Geometry check sheet. Reference: the model listing, model coordinates, mm. Coordinates: 2 decimals unless noted, no trailing zeros. One line per item, written item: value.
Autodesk Inventor part; units mm, degrees
ref_plane "YZ Plane" through (0, 0, 0) normal (1, 0, 0) x (0, 1, 0)
ref_plane "XZ Plane" through (0, 0, 0) normal (0, 1, 0) x (-1, 0, 0)
ref_plane "XY Plane" through (0, 0, 0) normal (0, 0, 1) x (1, 0, 0)
sketch "T-Slot 4040 Base" plane through (0, 0, 0) normal (0, 0, 1) x (1, 0, 0)
  line L0 (-28, 0) -> (28, 0) construction
  line L1 (0, -28) -> (0, 28) construction
  circle A0 centre (0, 0) radius 5.1
  line L2 (-7.5, -7.5) -> (7.5, -7.5)
  line L3 (7.5, -7.5) -> (7.5, 7.5)
  line L4 (7.5, 7.5) -> (-7.5, 7.5)
  line L5 (-7.5, 7.5) -> (-7.5, -7.5)
  line L6 (-7.5, -7.5) -> (7.5, 7.5) construction
  line L7 (7.5, -7.5) -> (-7.5, 7.5) construction
  line L8 (-20, 20) -> (20, 20)
  line L9 (20, 20) -> (20, -20)
  line L10 (20, -20) -> (-20, -20)
  line L11 (-20, -20) -> (-20, 20)
  line L12 (-20, 20) -> (20, -20) construction
  line L13 (20, 20) -> (-20, -20) construction
  line L14 (20, 5) -> (14.5, 5)
  line L15 (14.5, 5) -> (14.5, 10)
  line L16 (14.5, 10) -> (12.4749, 10)
  line L17 (12.4749, 10) -> (7.5, 5.0251)
  line L18 (5, 20) -> (5, 14.5)
  line L19 (5, 14.5) -> (10, 14.5)
  line L20 (10, 14.5) -> (10, 12.4749)
  line L21 (10, 12.4749) -> (5.0251, 7.5)
  line L22 (18.5, 18.5) -> (11.5, 18.5)
  line L23 (11.5, 18.5) -> (11.5, 11.5)
  line L24 (11.5, 11.5) -> (18.5, 11.5)
  line L25 (18.5, 11.5) -> (18.5, 18.5)
  line L26 (18.5, 18.5) -> (11.5, 11.5) construction
  line L27 (11.5, 18.5) -> (18.5, 11.5) construction
  line L28 (3.0732, 1.3088) -> (4.38, 2.6125) construction
  line L29 (5.905, 4.1338) -> (4.1393, 5.9037)
  line L30 (4.1393, 5.9037) -> (2.6122, 4.3802)
  line L31 (1.3075, 3.0787) -> (3.0732, 1.3088) construction
  line L32 (3.0732, 1.3088) -> (4.1393, 5.9037) construction
  line L33 (5.905, 4.1338) -> (1.3075, 3.0787) construction
  line L34 (4.38, 2.6125) -> (5.905, 4.1338)
  line L35 (2.6122, 4.3802) -> (1.3075, 3.0787) construction
  line L36 (-20, 5) -> (-14.5, 5)
  line L37 (-14.5, 5) -> (-14.5, 10)
  line L38 (-14.5, 10) -> (-12.4749, 10)
  line L39 (-12.4749, 10) -> (-7.5, 5.0251)
  line L40 (-5, 20) -> (-5, 14.5)
  line L41 (-5, 14.5) -> (-10, 14.5)
  line L42 (-10, 14.5) -> (-10, 12.4749)
  line L43 (-10, 12.4749) -> (-5.0251, 7.5)
  line L44 (-18.5, 18.5) -> (-11.5, 18.5)
  line L45 (-11.5, 18.5) -> (-11.5, 11.5)
  line L46 (-11.5, 11.5) -> (-18.5, 11.5)
  line L47 (-18.5, 11.5) -> (-18.5, 18.5)
  line L48 (-5.905, 4.1338) -> (-4.1393, 5.9037)
  line L49 (-4.1393, 5.9037) -> (-2.6122, 4.3802)
  line L50 (-4.38, 2.6125) -> (-5.905, 4.1338)
  line L51 (7.5, -7.5) -> (-7.5, -7.5)
  line L52 (20, -5) -> (14.5, -5)
  line L53 (14.5, -5) -> (14.5, -10)
  line L54 (14.5, -10) -> (12.4749, -10)
  line L55 (12.4749, -10) -> (7.5, -5.0251)
  line L56 (5, -20) -> (5, -14.5)
  line L57 (5, -14.5) -> (10, -14.5)
  line L58 (10, -14.5) -> (10, -12.4749)
  line L59 (10, -12.4749) -> (5.0251, -7.5)
  line L60 (18.5, -18.5) -> (11.5, -18.5)
  line L61 (11.5, -18.5) -> (11.5, -11.5)
  line L62 (11.5, -11.5) -> (18.5, -11.5)
  line L63 (18.5, -11.5) -> (18.5, -18.5)
  line L64 (18.5, -18.5) -> (11.5, -11.5) construction
  line L65 (11.5, -18.5) -> (18.5, -11.5) construction
  line L66 (3.0732, -1.3088) -> (4.38, -2.6125) construction
  line L67 (5.905, -4.1338) -> (4.1393, -5.9037)
  line L68 (4.1393, -5.9037) -> (2.6122, -4.3802)
  line L69 (1.3075, -3.0787) -> (3.0732, -1.3088) construction
  line L70 (3.0732, -1.3088) -> (4.1393, -5.9037) construction
  line L71 (5.905, -4.1338) -> (1.3075, -3.0787) construction
  line L72 (4.38, -2.6125) -> (5.905, -4.1338)
  line L73 (2.6122, -4.3802) -> (1.3075, -3.0787) construction
  line L74 (-4.38, -2.6125) -> (-5.905, -4.1338)
  line L75 (-4.1393, -5.9037) -> (-2.6122, -4.3802)
  line L76 (-5.905, -4.1338) -> (-4.1393, -5.9037)
  line L77 (-12.4749, -10) -> (-7.5, -5.0251)
  line L78 (-10, -12.4749) -> (-5.0251, -7.5)
  line L79 (-10, -14.5) -> (-10, -12.4749)
  line L80 (-5, -14.5) -> (-10, -14.5)
  line L81 (-5, -20) -> (-5, -14.5)
  line L82 (-18.5, -18.5) -> (-11.5, -18.5)
  line L83 (-11.5, -18.5) -> (-11.5, -11.5)
  line L84 (-11.5, -11.5) -> (-18.5, -11.5)
  line L85 (-18.5, -11.5) -> (-18.5, -18.5)
  line L86 (-14.5, -10) -> (-12.4749, -10)
  line L87 (-14.5, -5) -> (-14.5, -10)
  line L88 (-20, -5) -> (-14.5, -5)
  point P0 (15, 15)
  point P1 (3.6062, 3.6062)
  point P2 (3.6062, 3.6062)
  point P3 (15, -15)
  point P4 (3.6062, -3.6062)
  point P5 (3.6062, -3.6062)
  dimension "d9" = 10.2
  dimension "d12" = 40
  dimension "d13" = 40
  dimension "d14" = 5.5
  dimension "d15" = 15
  dimension "d16" = 7
  dimension "d17" = 10
  dimension "d20" = 1.75
  dimension "d21" = 7
  dimension "d22" = 2
  dimension "d29" = 1.5
  dimension "d30" = 2.5
extrude "Extrusion1" add sketch "T-Slot 4040 Base" along normal blind 500 contours L5 L4 L3 L2 | L2 L78 L79 L80 L81 L10 L11 L88 L87 L86 L77 L5 | L2 L3 L55 L54 L53 L52 L9 L10 L56 L57 L58 L59 | L39 L38 L37 L36 L11 L8 L40 L41 L42 L43 L4 L5 | L3 L4 L21 L20 L19 L18 L8 L9 L14 L15 L16 L17
fillet "Rundung1" radius 1 16 edges at (11.5, 18.5, 250) (18.5, 18.5, 250) (18.5, 11.5, 250) (11.5, 11.5, 250) (-11.5, 18.5, 250) (-18.5, 18.5, 250) (-18.5, 11.5, 250) (-11.5, 11.5, 250) (-18.5, -11.5, 250) (-11.5, -11.5, 250) (-11.5, -18.5, 250) (-18.5, -18.5, 250) (11.5, -18.5, 250) (11.5, -11.5, 250) (18.5, -11.5, 250) (18.5, -18.5, 250)
fillet "Rundung2" radius 3 4 edges at (20, 20, 250) (20, -20, 250) (-20, -20, 250) (-20, 20, 250)
properties part number "T-SLOT 4040 B-Type 500mm"
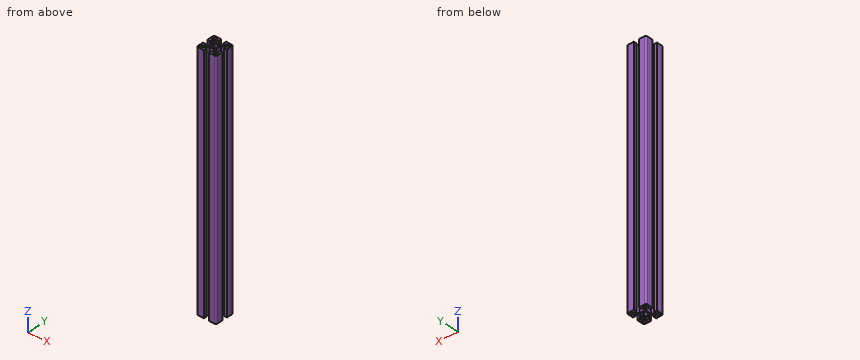
(1) Cross-section at A-A on z = 404.5. State how many separate pieces and enclosed holes the cut face has, and give its area (3 significant figures).
Reply:
separate pieces: 1
enclosed holes: 5
area: 616 mm2
(2) Material ranges on probe 1 along X at (y, z) = (17, 120.5); probe 2 along X at (y, z) = (12.5, 82), recorded low to high. Write a range as from..to.
Reply:
probe 1: -20..-18.5, -11.5..-5, 5..11.5, 18.5..20
probe 2: -20..-18.5, -11.5..-10, 10..11.5, 18.5..20
(3) Go/stop test with a flat-tipped pin: pin 1 Ø5 at (x, z) = (0, 259.5) entering from -Y. Record where the tip stops, or that it passes through.
Reply:
pin 1: y = -7.5
